from build123d import *

# Parameters (mm, degrees)
SKETCH1_W           = 50
SKETCH1_H           = 21.45
BOSS_EXTRUDE1_DEPTH = 6.5
SKETCH2_R           = 2.4
BOSS_EXTRUDE2_DEPTH = 10


with BuildPart() as part:
    # Sketch1 → Boss-Extrude1 (new body)
    with BuildSketch(Plane(origin=(0, 0, 0), x_dir=(1, 0, 0), z_dir=(0, 1, 0))):
        with Locations((25, 10.725)):
            Rectangle(SKETCH1_W, SKETCH1_H)
    extrude(amount=BOSS_EXTRUDE1_DEPTH)

    # Sketch2 → Boss-Extrude2 (add)
    with BuildSketch(Plane(origin=(50, 0, 0), x_dir=(0, 0, -1), z_dir=(1, 0, 0))):
        with Locations((10.725, 3.25)):
            Circle(SKETCH2_R)
        with Locations(Location((2.4, 3.25, 0), (0, 0, 180))):
            Circle(SKETCH2_R)
        with Locations((19.05, 3.25)):
            Circle(SKETCH2_R)
    extrude(amount=BOSS_EXTRUDE2_DEPTH)


solid = part.part
Input: part model. Units: mm. Frame: model coordinates. A direction names the side the tool comes from. Coordinates: 2 decimals unless noted, no trailing zeros. Write each loop counter-clockwise with the first axis right and the second up, starting at its lowest first coordinate (ties: lowest second). Pieces come first, ordered by that corner, then holes. Notation, with made-up numbers: M 18,-30.5 L 55,-30.5 A35 cw 55,8.5 Z; hole C 15.25,58 d1. An arc over 180 degrees is marked long. Answer as a JSON object with one key per item and string values. Group by question number.
(1) Ray query, line 1 along Z through (x, y) = (53, 3); line 2 along X through (y, z) = (0.75, -2.75); line 3 along Z through (x, y) = (56, 4.5). Return the intervals inside material, ascending. Write a range as [from, to].
(2) Section C-C on y = 2. Output: boundary loops of the cut face in (x, z).
(3) Section B-B on x = 53. Output: boundary loops of the cut face in (y, z) (3 decimals).
(4) Set-up query: faces 1 (the face through (25, 6.5, -11)), 2 (the face through (50, 3, -8)). Return all of +Z, -Z, +X, -X, +Y, -Y with unobstructed straight access to the full face (end or side cutting, diameter ignored); none if empty.
(5) Section D-D on z = -19.25. Output: boundary loops of the cut face in (x, y).
(6) Section A-A on z = -2.4. Output: boundary loops of the cut face in (x, y).
(7) Mould query, pull axis Z, two halves, no side actions, for faces 3 (the face through (54.93, 3.144, -4.798)), 4 (the face through (25, 3, -21.45)), 5 (the face through (25, 0, -11)), 6 (the face through (54.93, 3.356, -16.652)). Classes: pulls with the +Z half, pulls with the -Z half, needs draft (parallel to the pull), parting line crosses it, or undercut.
Result set:
{
 "1": {"line 1": "z = [-21.44, -16.66], [-13.11, -8.34], [-4.79, -0.01]", "line 2": "x = [0, 50]", "line 3": "z = [-21.1, -17], [-12.77, -8.68], [-4.45, -0.35]"},
 "2": {"outline": "M 0,-21.45 L 50,-21.45 L 50,-21.1 L 60,-21.1 L 60,-17 L 50,-17 L 50,-12.77 L 60,-12.77 L 60,-8.68 L 50,-8.68 L 50,-4.45 L 60,-4.45 L 60,-0.35 L 50,-0.35 L 50,0 L 0,0 Z"},
 "3": {"outline": "C 3.25,-19.05 d4.8; C 3.25,-10.725 d4.8; C 3.25,-2.4 d4.8"},
 "4": {"face 1": "+Z, -Z, +X, -X, +Y", "face 2": "+X"},
 "5": {"outline": "M 0,0 L 50,0 L 50,0.86 L 60,0.86 L 60,5.64 L 50,5.64 L 50,6.5 L 0,6.5 Z"},
 "6": {"outline": "M 0,0 L 50,0 L 50,0.85 L 60,0.85 L 60,5.65 L 50,5.65 L 50,6.5 L 0,6.5 Z"},
 "7": {"face 3": "undercut", "face 4": "pulls with the -Z half", "face 5": "needs draft", "face 6": "undercut"}
}
